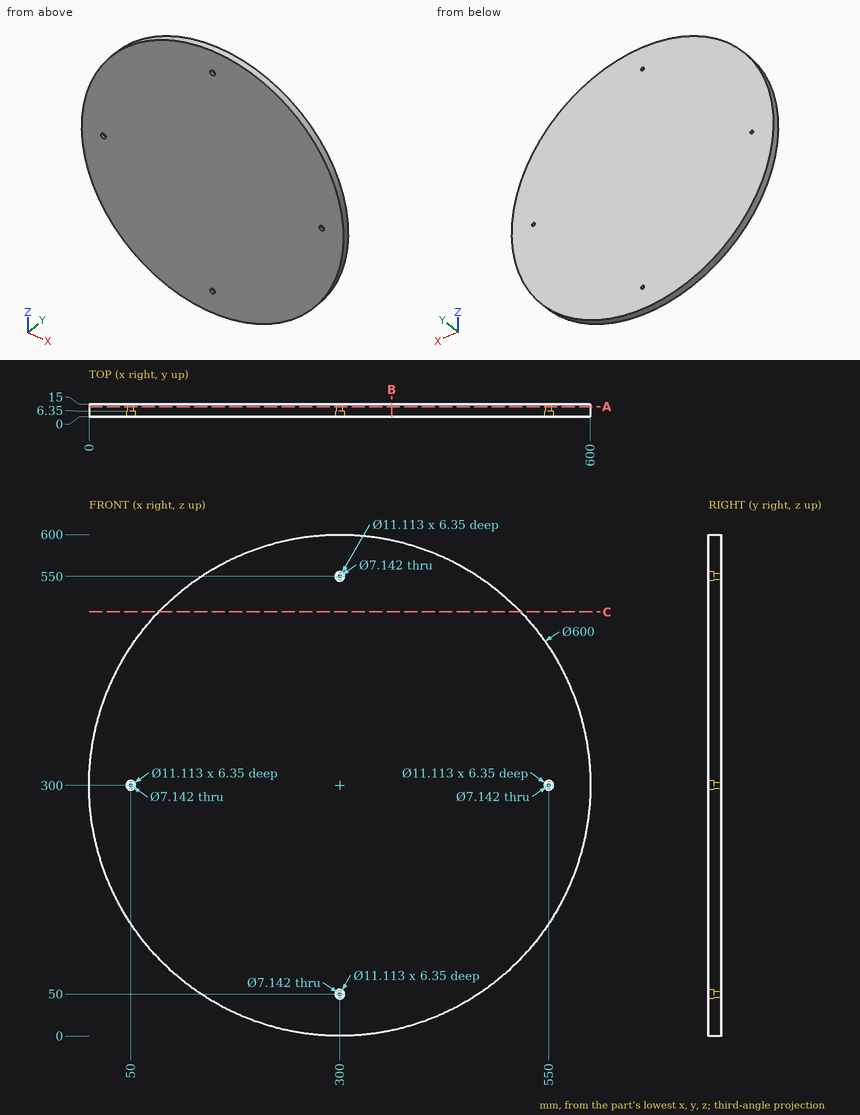
Input: dimensioned drawing with shaded views. Units: mm. Origin: part minimum x, y, z. Round coordinates to 2 decimals unless told otherwise and drop trailing zeros. Order: outer loops, then holes, each group sorted by start corner. A loop starts at its lowest first (then second) coordinate and runs counter-clockwise, first axis right, second up. Notation, with made-up numbers: (34, -18.75) - (78, -18.75) arc R13 ccw to (78, -8.75) - close; hole circle Ø6 at (79, 52). An arc over 180 degrees is marked (long way). Write item = value, one per line. Start each with the question number.
Q1. Ray query, line 1 (X direction, y = 3, z = 300); line 2 (X direction, y = 10.75, z = 50) (1 decimal). Return the intervals inside material, ascending. Write a range as from..to.
Q2. Cut plane B-B on x = 362. Return the cut outline in (y, z).
Q3. Cut plane C-C on z = 507.5. Return the cut outline in (x, y) (1 decimal), and give its area (3 significant figures).
Q4. Pin query (flat end, axial travel): pin 1 (4.5 mm diameter, centred on x = 300, z = 550, fed in from -Y); pin 2 (8 mm diameter, centred on x = 391.5, y = 12, fed in from -Z); pin 3 (5.5 mm diameter, centred on x = 297.5, z = 549, fed in from -Y); pin 4 (2 mm diameter, centred on x = 105.5, y = 8, fed in from -Z) (1 decimal). Return the tip coordinate at first contact, or that it passes through.
Q5. Cut plane A-A on y = 11.75. Return the cut outline in (x, z).
Outcome:
q1.line_1 = 0..44.44, 55.56..544.44, 555.56..600
q1.line_2 = 134.2..296.4, 303.6..465.8
q2.outline = (0, 6.48) - (15, 6.48) - (15, 593.52) - (0, 593.52) - close
q3.outline = (83.3, 0) - (516.7, 0) - (516.7, 15) - (83.3, 15) - close
q3.area = 6,500 mm^2
q4.pin_1 = through
q4.pin_2 = 13.04
q4.pin_3 = 6.35
q4.pin_4 = 70.7
q5.outline = circle Ø600 at (300, 300); hole circle Ø7.14 at (50, 300); hole circle Ø7.14 at (300, 50); hole circle Ø7.14 at (300, 550); hole circle Ø7.14 at (550, 300)
